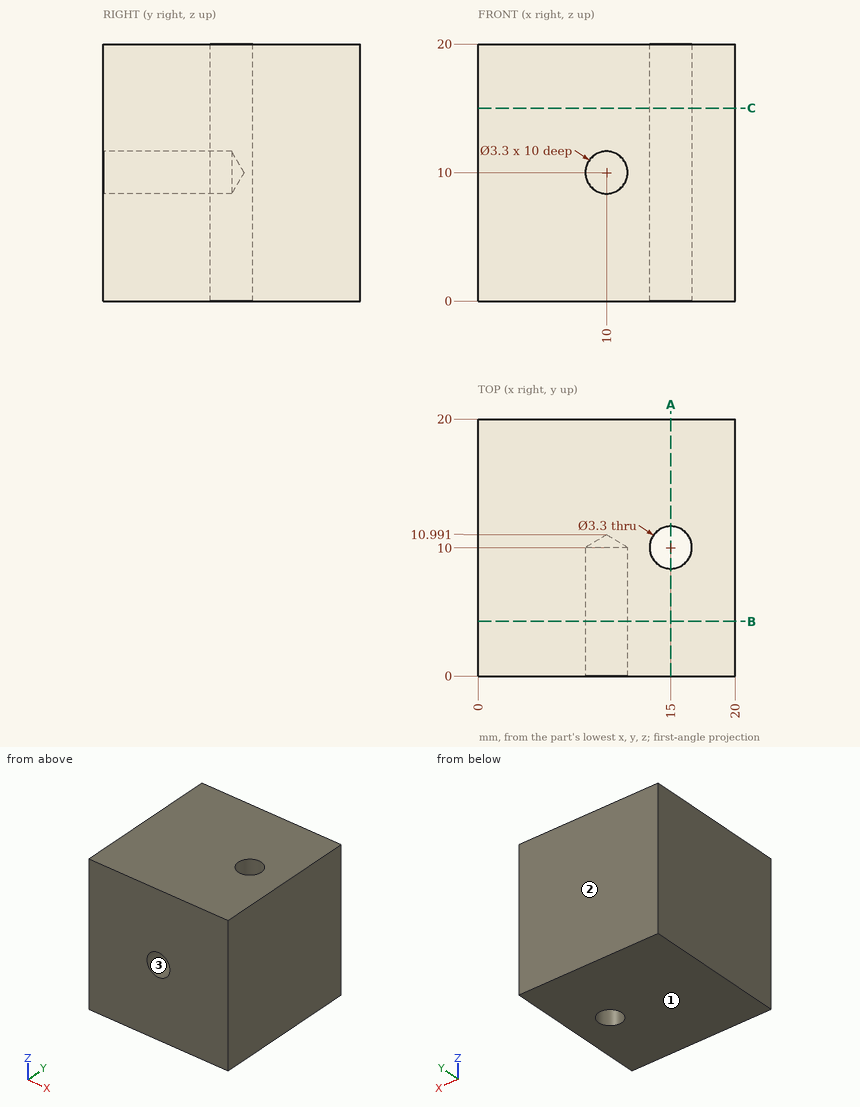
The figure shows three views and two pictorial views of one solid part (mm, origin at its lowest corner). Answer the questions. Give positions to 0.01 mm unless a question says otherwise; leave off trailing zeros. Loops run counter-clockwise (first coordinate to the right, second up) from the corner with the lowest first, then second, coordinate; pieces in that order, holes last. Notation, with made-up numbers: M -5,4.25 L 15,4.25 A20 cw 15,28.25 Z; hole C 59.25,57.5 d3. An arc over 180 degrees is marked long. Write each question's results on one line, items separated by ' | '.
1. Section C-C on z = 15 is taken. Give the vertices of the cut face in (x, y).
Values:
outline: M 0,0 L 20,0 L 20,20 L 0,20 Z; hole C 15,10 d3.3
2. Section A-A on x = 15 is taken. Give the vertices of the cut face in (y, z).
Values:
outline: M 0,0 L 8.35,0 L 8.35,20 L 0,20 Z; M 11.65,0 L 20,0 L 20,20 L 11.65,20 Z
3. Given pin 1 (3 mm diameter, centred on x = 10, z = 10, fed in from -Y), flat-ended and moving along its own axis, determine where the tip first touches the part or whether it passes through.
Values:
pin 1: stops at y = 10.09
4. Section B-B on y = 4.25 is taken. Give the vertices of the cut face in (x, z).
Values:
outline: M 0,0 L 20,0 L 20,20 L 0,20 Z; hole C 10,10 d3.3
5. Straight lines are drawn through the part: line 1 (Z direction, x = 10, y = 5.75); line 2 (Z direction, x = 11, y = 9); line 3 (X direction, y = 11, z = 2.5). For each, find the intervals that lie inside material, in ascending order. Write a range as [from, to].
Values:
line 1: z = [0, 8.35], [11.65, 20] | line 2: z = [0, 8.69], [11.31, 20] | line 3: x = [0, 13.69], [16.31, 20]
6. The mould has two halves that part along Z. Classify the marked faces 1, 2 and 3: pulls with the +Z half, pulls with the -Z half, needs draft (parallel to the pull), parting line crosses it, or undercut.
Values:
face 1: pulls with the -Z half | face 2: needs draft | face 3: undercut
